from build123d import *

# Parameters (mm, degrees)
IZIM1_W                          = 55
IZIM1_H                          = 18
Y_KSEKLIK_EKSTR_ZYON1_DEPTH      = 10
KES_EKSTR_ZYON1_DEPTH            = 59.72818744
IZIM3_R                          = 6
Y_KSEKLIK_EKSTR_ZYON2_DEPTH      = 100
IZIM5_W                          = 12
IZIM5_H                          = 12
Y_KSEKLIK_EKSTR_ZYON3_DEPTH      = 12
IZIM7_R                          = 0.75
KES_EKSTR_ZYON3_DEPTH            = 131.929342088
Y_KSEKLIK_EKSTR_ZYON4_DEPTH      = 34
Y_KSEKLIK_EKSTR_ZYON4_DEPTH_BACK = 80
IZIM6_R                          = 8.485281374


with BuildPart() as part:
    # Çizim1 → Yükseklik-Ekstrüzyon1 (new body)
    with BuildSketch(Plane(origin=(0, 0, 0), x_dir=(1, 0, 0), z_dir=(0, 1, 0))):
        with Locations((27.5, -9)):
            Rectangle(IZIM1_W, IZIM1_H)
    extrude(amount=-Y_KSEKLIK_EKSTR_ZYON1_DEPTH)

    # Çizim2 → Kes-Ekstrüzyon1 (cut, through all)
    with BuildSketch(Plane.ZY):
        Polygon((18, -10), (0, -2.63065823), (0, -10), align=None)
    extrude(amount=-KES_EKSTR_ZYON1_DEPTH, mode=Mode.SUBTRACT)

    # Çizim3 → Yükseklik-Ekstrüzyon2 (add)
    with BuildSketch(Plane(origin=(0, -2.253018898, -0.922403682), x_dir=(-1, 0, 0), z_dir=(0, -0.9254441249587121, -0.3788841136540354))):
        with Locations(Location((-10, -10.721774999, 0), (0, 0, 270))):
            Circle(IZIM3_R)
        with Locations(Location((-44.231710038, -10.721774999, 0), (0, 0, 270))):
            Circle(IZIM3_R)
    extrude(amount=Y_KSEKLIK_EKSTR_ZYON2_DEPTH)

    # Çizim5 → Yükseklik-Ekstrüzyon3 (add)
    with BuildSketch(Plane(origin=(0, -94.797431394, -38.810815047), x_dir=(-1, 0, 0), z_dir=(0, -0.9254441249587119, -0.37888411365403546))):
        with Locations((-10, -10.721774999)):
            Rectangle(IZIM5_W, IZIM5_H)
        with Locations((-44.231710038, -10.721774999)):
            Rectangle(IZIM5_W, IZIM5_H)
    extrude(amount=Y_KSEKLIK_EKSTR_ZYON3_DEPTH)

    # Çizim7 → Kes-Ekstrüzyon3 (cut, through all)
    with BuildSketch(Plane(origin=(0, 0, 0), x_dir=(1, 0, 0), z_dir=(0, 1, 0))):
        with Locations(Location((2.5, -9, 0), (0, 0, 270))):
            Circle(IZIM7_R)
        with Locations(Location((52.5, -9, 0), (0, 0, 270))):
            Circle(IZIM7_R)
    extrude(amount=-KES_EKSTR_ZYON3_DEPTH, mode=Mode.SUBTRACT)

    # Çizim6 → Yükseklik-Ekstrüzyon4 (add, two sides: drawn at the far end of the back side and taken through both)
    with BuildSketch(Plane.ZY.offset(-4).offset(-Y_KSEKLIK_EKSTR_ZYON4_DEPTH_BACK)):
        with Locations((-31.161716047, -104.412406361)):
            Circle(IZIM6_R)
    extrude(amount=Y_KSEKLIK_EKSTR_ZYON4_DEPTH + Y_KSEKLIK_EKSTR_ZYON4_DEPTH_BACK)


solid = part.part
For this review, take the finished solid that the model builds, in its own axes (mm). A direction names the side the tool comes from. Give positions to 0.01 mm unless a question says otherwise; leave off trailing zeros. Loops run counter-clockwise (first coordinate to the right, second up) from the corner with the lowest first, then second, coordinate; pieces in that order, holes last. Notation, with made-up numbers: M 76.25,-15.5 L 124.25,-15.5 A18 ccw 124.25,-11.5 Z; hole C 3.5,33 d5. An arc over 180 degrees is marked long. Put each result on its own line as item: value. Start each with the question number.
(1) Wall thickness on L1, parallel to X at y = -3.5, z = 9; L2, parallel to Z at x = 2.5, y = -1.5; L3, parallel to X at y = -94, z = -25.5: over which ranges is each line inside the solid? List them lowest first.
(2) Add section B-B, the plane x = -5. Write out the cut boundary in (y, z), then the cut area to 3 significant figures.
(3) For pin 1 (8 mm diameter, centred on x = 69, z = -25, fed in from -Y); pin 2 (2 mm diameter, centred on y = -88, z = -27, fed in from -X); pin 3 (3 mm diameter, centred on y = -3.5, z = 10, fed in from -X); pin 4 (2.5 mm diameter, centred on x = 2.5, z = 9, fed in from +Y), all flat-tipped, find the tip position at first contact; note any pin that passes through.
(4) Add section A-A, the plane x = 28. Write out the cut boundary in (y, z).
(5) Machinability: for faces 1 (the flat face through (27, 0, 9)), 2 (the flat face through (27, -1, 0)), which of the approach directions +Z, -Z, +X, -X, +Y, -Y give a long, thin tool a straight path to every point of the face, cutting with its end or side? Answer none if there is none.
(6) The part is to be moulded in two halves that separate along X. For faces 3 (the flat face through (84, -104, -31)), 4 (the cylindrical face through (15.86, -51.45, -10.88)), 5 (the flat face through (0, -4, 11)), 6 (the flat face through (27.12, -6.37, 9.13)), say which applies: +X half, -X half, draft (parallel to the pull), parting line (faces both ways), or undercut.
Result:
1. L1: x = 0 to 1.75, 3.25 to 51.75, 53.25 to 55
1. L2: z = 0 to 8.25, 9.75 to 18
1. L3: x = 4.14 to 15.86, 38.37 to 50.09
2. outline: C -104.41,-31.16 d16.97
2. area: 226 mm^2
3. pin 1: stops at y = -112.62
3. pin 2: stops at x = 4.16
3. pin 3: stops at x = 0
3. pin 4: stops at y = 0
4. outline: C -104.41,-31.16 d16.97; M -10,18 L -2.63,0 L 0,0 L 0,18 Z
5. face 1: +Z, -Z, +X, -X, +Y
5. face 2: -Z, +X, -X, +Y
6. face 3: +X half
6. face 4: undercut
6. face 5: -X half
6. face 6: undercut
